Check sheet for the modelled part. Datum: model origin and axes. Units: mm. Face numbers are marked on the shaded views. A direction names the side the tool comes from. Coordinates: 2 decimals unless noted, no trailing zeros. Loops run counter-clockwise (first coordinate to the right, second up) from the corner with the lowest first, then second, coordinate; pieces in that order, holes last. Notation, with made-up numbers: M -20.5,17.5 L 18.5,17.5 A14 cw 18.5,41.5 Z; hole C 75.25,-22 d3. An arc over 180 degrees is marked long. Return JSON: item names as keys, results as strings.
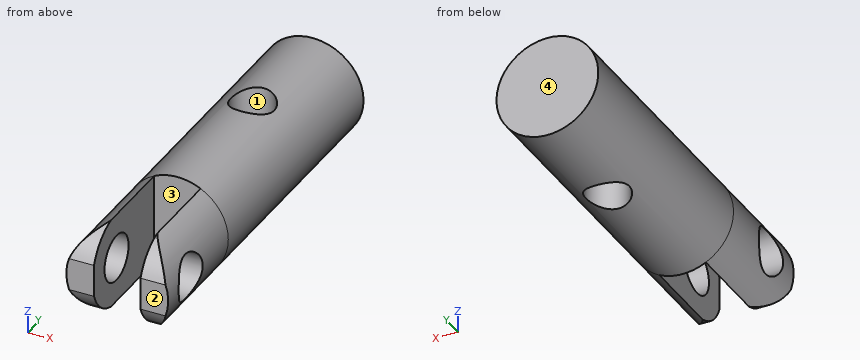
from build123d import *

# Parameters (mm, degrees)
SKETCH1_R               = 8.75
BOSS_EXTRUDE1_DEPTH     = 45
BOSS_EXTRUDE2_DEPTH     = 20
SKETCH3_R               = 4
CUT_EXTRUDE2_DEPTH      = 15
CUT_EXTRUDE2_DEPTH_BACK = 15
SKETCH4_R               = 3.75
CUT_EXTRUDE3_DEPTH      = 15
CUT_EXTRUDE3_DEPTH_BACK = 15


with BuildPart() as part:
    # Sketch1 → Boss-Extrude1 (new body)
    with BuildSketch(Plane(origin=(0, 0, 0), x_dir=(1, 0, 0), z_dir=(0, 1, 0))):
        Circle(SKETCH1_R)
    extrude(amount=BOSS_EXTRUDE1_DEPTH)

    # Sketch2 → Boss-Extrude2 (add)
    with BuildSketch(Plane.XZ):
        with BuildLine():
            Line((-4, -7.782191), (-4, 7.782191))
            ThreePointArc((-4, 7.782191), (-8.75, 0), (-4, -7.782191))
        make_face()
        with BuildLine():
            Line((4, -7.782191), (4, 7.782191))
            ThreePointArc((4, 7.782191), (8.75, 0), (4, -7.782191))
        make_face()
    extrude(amount=BOSS_EXTRUDE2_DEPTH)

    # Sketch3 → Cut-Extrude2 (cut, two sides)
    with BuildSketch(Plane(origin=(0, 0, 0), x_dir=(0, 0, -1), z_dir=(1, 0, 0))) as cut_extrude2_sk:
        with Locations((0, -12.5)):
            Circle(SKETCH3_R)
        with BuildLine():
            Line((-8, -12.5), (-11.944744, -12.5))
            Line((-11.944744, -12.5), (-11.944744, -23.565323))
            Line((-11.944744, -23.565323), (12.069953, -23.565323))
            Line((12.069953, -23.565323), (12.069953, -12.5))
            Line((12.069953, -12.5), (8, -12.5))
            ThreePointArc((8, -12.5), (0, -20.5), (-8, -12.5))
        make_face()
    extrude(amount=CUT_EXTRUDE2_DEPTH, mode=Mode.SUBTRACT)
    extrude(cut_extrude2_sk.sketch, amount=-CUT_EXTRUDE2_DEPTH_BACK, mode=Mode.SUBTRACT)

    # Sketch4 → Cut-Extrude3 (cut, two sides)
    with BuildSketch(Plane.XY) as cut_extrude3_sk:
        with Locations((0, 25)):
            Circle(SKETCH4_R)
    extrude(amount=CUT_EXTRUDE3_DEPTH, mode=Mode.SUBTRACT)
    extrude(cut_extrude3_sk.sketch, amount=-CUT_EXTRUDE3_DEPTH_BACK, mode=Mode.SUBTRACT)


solid = part.part
1) Section check D-D on y = -2.5. Record the cut outline in (x, z), then the cut area to 3 significant figures.
Answers:
{"outline": "M -4,-7.78 L -4,7.78 A8.75 ccw Z; M 4,-7.78 A8.75 ccw 4,7.78 Z", "area": "106 mm²"}
2) Section check A-A on z = 0. Record the cut outline in (x, y), then the cut area to 3 significant figures.
Answers:
{"outline": "M -8.75,-20 L -4,-20 L -4,-16.5 L -8.75,-16.5 Z; M -8.75,-8.5 L -4,-8.5 L -4,0 L 4,0 L 4,-8.5 L 8.75,-8.5 L 8.75,45 L -8.75,45 Z; M 4,-20 L 8.75,-20 L 8.75,-16.5 L 4,-16.5 Z; hole C 0,25 d7.5", "area": "857 mm²"}
3) Set-up check for the marked faces 3 and 4: record each of +Z, -Z, +X, -X, +Y, -Y from which the full face is reachable in a straight line by a thin tool's end or side.
Answers:
{"face 3": "+Z, -Z, -Y", "face 4": "+Z, -Z, +X, -X, +Y"}
4) Draft check along X on the marked faces 1 and 2. Enter one of: +X half, -X half, draft (parallel to the pull), parting line (faces both ways), or undercut.
Answers:
{"face 1": "undercut", "face 2": "draft"}
5) Section check C-C on y = -12.5. Record the cut outline in (x, z).
Answers:
{"outline": "M -7.78,-4 A8.75 ccw -4,-7.78 L -4,-4 Z; M -7.78,4 L -4,4 L -4,7.78 A8.75 ccw Z; M 4,-7.78 A8.75 ccw 7.78,-4 L 4,-4 Z; M 4,4 L 7.78,4 A8.75 ccw 4,7.78 Z"}
6) Scan lines: line 1 along Y through (x, z) = (0, 2.25); line 2 along Y through (x, z) = (-6.15, 0); line 3 along X through (y, z) = (-17, 2.5). Record each from-to range of solid material in increasing order. Write a range as [from, to].
Answers:
{"line 1": "[0, 21.25], [28.75, 45]", "line 2": "[-20, -16.5], [-8.5, 45]", "line 3": "[-8.39, -4], [4, 8.39]"}
7) Go/stop test with flat-tipped pins: pin 1 Ø4.5 at (y, z) = (-10, 2) entering from -X; pin 2 Ø8 at (y, z) = (-5.5, 3.5) entering from +X; pin 3 Ø6 at (x, y) = (-3.5, -11.5) entering from +Z; pin 4 Ø2 at (x, y) = (6, 14) entering from -Z. Record where each tip stops, or that it passes through.
Answers:
{"pin 1": "x = -8.74", "pin 2": "x = 8.75", "pin 3": "z = 7.78", "pin 4": "z = -7.18"}
8) Section check B-B on x = 0. Record the cut outline in (y, z).
Answers:
{"outline": "M 0,-8.75 L 21.25,-8.75 L 21.25,8.75 L 0,8.75 Z; M 28.75,-8.75 L 45,-8.75 L 45,8.75 L 28.75,8.75 Z"}
